Job drawing, mm, ordinate dimensions from the low corner. One solid piece. Coordinates: 2 decimals unless noted, no trailing zeros. Loops run counter-clockwise (first coordinate to the right, second up) from the corner with the lowest first, then second, coordinate; pieces in that order, holes last. Notation, with made-up numbers: M -7.5,26.25 L 38.5,26.25 A17 ccw 38.5,41.25 Z; hole C 79.5,-39.5 d9. An arc over 180 degrees is marked long. Answer as a JSON object with one key per item and string values. Group by question number.
1. Drill centre lines: L1, parallel to Z at x = 320, y = 43; L2, parallel to X at y = 100, z = 36.5; L3, parallel to Z at x = 81, y = 64 (1 decimal). Where is each one in solid material? Low to high.
2. Drop flat-ended pins along their axis: pin 1 Ø15 at (x, y) = (280, 100) entering from -Z; pin 2 Ø16.5 at (x, y) = (120, 100) entering from +Z (1 decimal); pin 3 Ø20.5 at (x, y) = (360, 100) entering from +Z; pin 4 Ø1 at (x, y) = (121.5, 27) entering from +Z. Give the stop position or say it passes through.
3. Mould opens along Z. For the marked faces 1, 2 and 3 say: released by +Z, released by -Z, zero draft, split by the parting line, or undercut.
4. Saw through at B-B on y = 41.5. Write the cut outline in (x, z).
5. Saw through at A-A on x = 360. Count the separate pieces of the cut face and the enclosed holes in it, then the cut area to 3 significant figures.
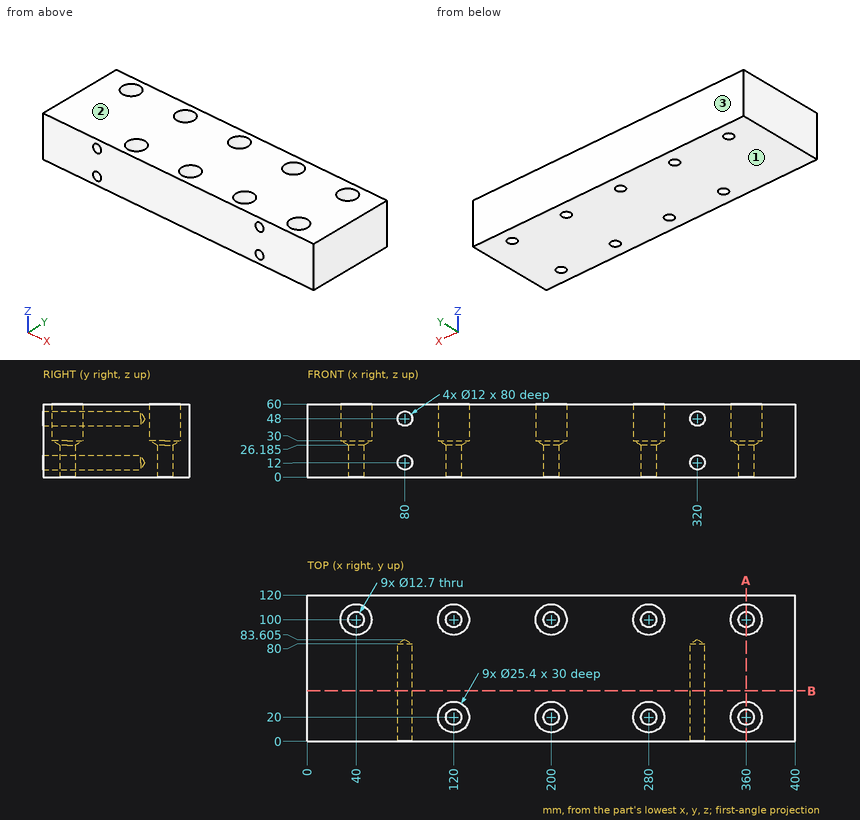
Outcome:
{
 "1": {"L1": "z = 0 to 6, 18 to 42, 54 to 60", "L2": "x = 0 to 27.3, 52.7 to 107.3, 132.7 to 187.3, 212.7 to 267.3, 292.7 to 347.3, 372.7 to 400", "L3": "z = 0 to 6.1, 17.9 to 42.1, 53.9 to 60"},
 "2": {"pin 1": "stops at z = 0", "pin 2": "stops at z = 27.3", "pin 3": "stops at z = 28.53", "pin 4": "stops at z = 26.97"},
 "3": {"face 1": "released by -Z", "face 2": "released by +Z", "face 3": "zero draft"},
 "4": {"outline": "M 0,0 L 400,0 L 400,60 L 0,60 Z; hole C 80,12 d12; hole C 80,48 d12; hole C 320,12 d12; hole C 320,48 d12"},
 "5": {"separate pieces": "3", "enclosed holes": "0", "area": "4,870 mm²"}
}
